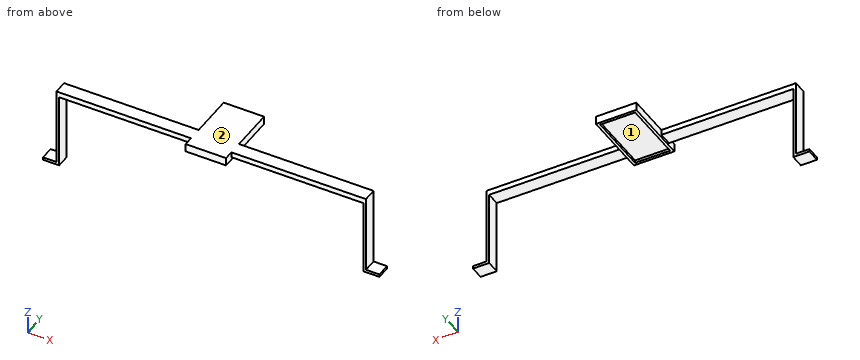
```python
from build123d import *

# Parameters (mm, degrees)
BOSS_EXTRUDE2_DEPTH = 5
SKETCH3_W           = 15
SKETCH3_H           = 25
SKETCH3_W_2         = 13
SKETCH3_H_2         = 23
BOSS_EXTRUDE3_DEPTH = 1
SKETCH5_W           = 15
SKETCH5_H           = 25
BOSS_EXTRUDE5_DEPTH = 2


with BuildPart() as part:
    # Sketch1 → Boss-Extrude2 (new body)
    with BuildSketch(Plane(origin=(0, 0, 0), x_dir=(1, 0, 0), z_dir=(0, 1, 0))):
        Polygon((-57.5, -1), (57.5, -1), (57.5, 28), (62.5, 28), (62.5, 29), (56.5, 29), (56.5, 1), (-56.5, 1), (-56.5, 29), (-62.5, 29), (-62.5, 28), (-57.5, 28), align=None)
    extrude(amount=BOSS_EXTRUDE2_DEPTH)

    # Sketch3 → Boss-Extrude3 (add)
    with BuildSketch(Plane(origin=(0, 0, -1), x_dir=(-1, 0, 0), z_dir=(0, 0, -1))):
        with Locations((0, 9)):
            Rectangle(SKETCH3_W, SKETCH3_H)
        with Locations((0, 9)):
            Rectangle(SKETCH3_W_2, SKETCH3_H_2, mode=Mode.SUBTRACT)
    extrude(amount=BOSS_EXTRUDE3_DEPTH)

    # Sketch5 → Boss-Extrude5 (add)
    with BuildSketch(Plane.XY.offset(-1)):
        with Locations((0, 9)):
            Rectangle(SKETCH5_W, SKETCH5_H)
    extrude(amount=BOSS_EXTRUDE5_DEPTH)


solid = part.part
```
Input: part model. Units: mm. Frame: model coordinates. Face numbers are marked on the shaded views. Coordinates: 2 decimals unless noted, no trailing zeros. Write each loop counter-clockwise with the first axis right and the second up, starting at its lowest first coordinate (ties: lowest second). Pieces come first, ordered by that corner, then holes. Notation, with made-up numbers: (-12.75, -14.75) -> (32.25, -14.75) arc R7 cw to (32.25, -6.75) -> close; hole circle Ø4 at (-20, 64). An arc over 180 degrees is marked (long way). Answer as a JSON object with one key per item and string values.
1. First-contact query: P1, Ø4, axis at y = 3, z = -18.5, coming from the +X side; P2, Ø4, axis at y = 0, z = -24, coming from the -X side; P3, Ø4, axis at x = 24, y = 2.5, coming from the -Z side; P4, Ø3, axis at x = -26.5, y = 8, coming from the +Z side. Flat tips, straight axial feed; report the tip coordinate or a pass-through.
Result set:
{"P1": "stops at x = 57.5", "P2": "stops at x = -57.5", "P3": "stops at z = -1", "P4": "passes through"}
2. Section D-D on x = 30. Return the cut outline in (y, z).
Result set:
{"outline": "(0, -1) -> (5, -1) -> (5, 1) -> (0, 1) -> close"}
3. Section A-A on z = -24.5. Return the cut outline in (x, y).
Result set:
{"outline": "(-57.5, 0) -> (-56.5, 0) -> (-56.5, 5) -> (-57.5, 5) -> close; (56.5, 0) -> (57.5, 0) -> (57.5, 5) -> (56.5, 5) -> close"}
4. Material intervals for line 1 (X direction, y = 9.25, z = -1.25); line 2 (Y direction, x = -57, z = -7.25); line 3 (Z direction, x = 0, y = 4.5), sorted ascending. Write a range as from..to.
Result set:
{"line 1": "x = -7.5..-6.5, 6.5..7.5", "line 2": "y = 0..5", "line 3": "z = -1..1"}
5. Section B-B on y = 8.75. Return the cut outline in (x, z), then the cut area to 3 significant figures.
Result set:
{"outline": "(-7.5, -2) -> (-6.5, -2) -> (-6.5, -1) -> (6.5, -1) -> (6.5, -2) -> (7.5, -2) -> (7.5, 1) -> (-7.5, 1) -> close", "area": "32.0 mm2"}
6. Mould query, pull axis X, two halves, no side actions, for the marked faces 1 and 2. Classes: released by +X, released by -X, zero draft, split by the parting line, or undercut.
Result set:
{"face 1": "undercut", "face 2": "zero draft"}
7. Section C-C on x = 3. Return the cut outline in (y, z), then the cut area to 3 significant figures.
Result set:
{"outline": "(-3.5, -2) -> (-2.5, -2) -> (-2.5, -1) -> (20.5, -1) -> (20.5, -2) -> (21.5, -2) -> (21.5, 1) -> (-3.5, 1) -> close", "area": "52.0 mm2"}
